Read the model definition and answer for the solid it produces. Units are mm, in the model's axes. A direction names the side the tool comes from. Give positions to 0.01 mm unless a question says otherwise; leave off trailing zeros. Order: outer loops, then holes, each group sorted by start corner. A loop starts at its lowest first (then second) coordinate and runs counter-clockwise, first axis right, second up. Notation, with made-up numbers: (35.5, 16.5) - (42.5, 16.5) arc R23 ccw to (42.5, 44.5) - close; hole circle Ø6 at (41, 15). An arc over 180 degrees is marked (long way). Return JSON: item names as keys, results as strings.
```python
from build123d import *

# Parameters (mm, degrees)
CROQUIS1_R                 = 9.5
SALIENTE_EXTRUIR1_DEPTH    = 120
CROQUIS3_R                 = 5.5
SALIENTE_EXTRUIR2_DEPTH    = 10
CROQUIS4_R                 = 2.5
CORTAR_EXTRUIR1_DEPTH      = 110
CORTAR_EXTRUIR2_DEPTH      = 110
CORTAR_EXTRUIR2_DEPTH_BACK = 110
CROQUIS5_R                 = 1.5


with BuildPart() as part:
    # Croquis1 → Saliente-Extruir1 (new body)
    with BuildSketch(Plane(origin=(0, 0, 0), x_dir=(1, 0, 0), z_dir=(0, 1, 0))):
        with Locations(Location((0, 0, 0), (0, 0, 270))):
            Circle(CROQUIS1_R)
    extrude(amount=SALIENTE_EXTRUIR1_DEPTH)

    # Croquis2 → Cortar-Revoluci_n1 (revolve, cut)
    with BuildSketch(Plane.XY, mode=Mode.PRIVATE) as cortar_revoluci_n1_sk:
        Polygon((-9.5, 22), (-9.5, 32), (-5.560768988, 21.305407289), align=None)
    revolve(cortar_revoluci_n1_sk.sketch.rotate(Axis((0, 120, 0), (0, -1, 0)), 270), axis=Axis((0, 120, 0), (0, -1, 0)), mode=Mode.SUBTRACT)

    # Croquis3 → Saliente-Extruir2 (add)
    with BuildSketch(Plane.XZ):
        with Locations(Location((0, 0, 0), (0, 0, 270))):
            Circle(CROQUIS3_R)
    extrude(amount=SALIENTE_EXTRUIR2_DEPTH)

    # Croquis4 → Cortar-Extruir1 (cut)
    with BuildSketch(Plane.XZ.offset(10)):
        with Locations(Location((0, 0, 0), (0, 0, 270))):
            Circle(CROQUIS4_R)
    extrude(amount=-CORTAR_EXTRUIR1_DEPTH, mode=Mode.SUBTRACT)

    # Croquis5 → Cortar-Extruir2 (cut, two sides: drawn at the far end of the back side and taken through both)
    with BuildSketch(Plane.XY.offset(-CORTAR_EXTRUIR2_DEPTH_BACK)):
        with Locations(Location((0, 95, 0), (0, 0, 180))):
            Circle(CROQUIS5_R)
    extrude(amount=CORTAR_EXTRUIR2_DEPTH + CORTAR_EXTRUIR2_DEPTH_BACK, mode=Mode.SUBTRACT)


solid = part.part
```
Q1. A cutting plane is placed at B-B (y = 95). Write down the section's boundary in (x, z).
Values:
{"outline": "(-1.5, -9.38) - (-1.5, -2) arc R2.5 cw to (-1.5, 2) - (-1.5, 9.38) arc R9.5 ccw to start; (1.5, -9.38) arc R9.5 ccw to (1.5, 9.38) - (1.5, 2) arc R2.5 cw to (1.5, -2) - close"}
Q2. For faces 1 (the conical face through (-1.99, 24.2, 6.32)), 2 (the cylindrical face through (1.5, 94.93, 5.7)), 3 (the flat face through (0, 100, 0)), determine the directions among +Z, -Z, +X, -X, +Y, -Y from which every point of the face is accessible in a straight line to the end or side of a thin tool.
Values:
{"face 1": "none", "face 2": "+Z, -Z", "face 3": "-Y"}
Q3. A cutting plane is placed at A-A (z = 7.25). Give the number of separate pieces and of enclosed holes in the cut face, and give its area (3 significant figures).
Values:
{"separate pieces": "2", "enclosed holes": "1", "area": "1,390 mm²"}
Q4. A cutting plane is placed at D-D (z = 0). Write down the section's boundary in (x, y), and give its area (3 significant figures).
Values:
{"outline": "(-9.5, 0) - (-5.5, 0) - (-5.5, -10) - (-2.5, -10) - (-2.5, 100) - (2.5, 100) - (2.5, -10) - (5.5, -10) - (5.5, 0) - (9.5, 0) - (9.5, 22) - (5.56, 21.31) - (9.5, 32) - (9.5, 120) - (-9.5, 120) - (-9.5, 32) - (-5.56, 21.31) - (-9.5, 22) - close", "area": "1,800 mm²"}
Q5. Given pin 1 (2 mm diameter, centred on y = 57.5, z = 5, fed in from +X); pin 2 (2 mm diameter, centred on x = -6.5, z = -5.5, fed in from -Y); pin 3 (5 mm diameter, centred on x = -5.5, y = 42, fed in from -Z); pin 4 (2.5 mm diameter, centred on x = 0, y = 95, fed in from -Z), each flat-ended and moving along its own axis, determine where each tip first touches the part or whether it passes through.
Values:
{"pin 1": "stops at x = 8.62", "pin 2": "stops at y = 0", "pin 3": "stops at z = -9.01", "pin 4": "passes through"}
Q6. Consider L1, parallel to Z at x = -0.25, y = 6.5; L2, parallel to X at y = 69, z = 0; L3, parallel to Y at x = 0, z = -3.5. Determine where each line is inside the solid, lowest interval first.
Values:
{"L1": "z = -9.5 to -2.49, 2.49 to 9.5", "L2": "x = -9.5 to -2.5, 2.5 to 9.5", "L3": "y = -10 to 93.5, 96.5 to 120"}
Q7. A cutting plane is placed at C-C (y = 60). Write down the section's boundary in (x, z).
Values:
{"outline": "circle Ø19 at (0, 0); hole circle Ø5 at (0, 0)"}
Q8. Determine the mould class of faces 4 (the flat face through (-4, 0, 4)), 5 (the cylindrical face through (-2.44, 44.23, 0.54)), 6 (the cylindrical face through (-5.37, -4.93, 1.19)) for opening direction Z: released by +Z, released by -Z, zero draft, split by the parting line, or undercut.
Values:
{"face 4": "zero draft", "face 5": "undercut", "face 6": "split by the parting line"}
